from build123d import *

# Parameters (mm, degrees)
SKETCH1_W               = 100
SKETCH1_H               = 40
BOSS_EXTRUDE1_DEPTH     = 5
CUT_EXTRUDE1_DEPTH      = 5
CUT_EXTRUDE2_DEPTH      = 5
CUT_EXTRUDE3_DEPTH      = 5
CUT_EXTRUDE4_DEPTH      = 5
SKETCH3_W               = 70
SKETCH3_H               = 25
BOSS_EXTRUDE2_DEPTH     = 100
FILLET1_R               = 5
FILLET2_R               = 2.5
CUT_EXTRUDE8_DEPTH      = 28.5
FILLET3_R               = 2.5
CUT_EXTRUDE9_DEPTH      = 8.077656227
CUT_EXTRUDE9_DEPTH_BACK = 38.464308309


with BuildPart() as part:
    # Sketch1 → Boss-Extrude1 (new body)
    with BuildSketch(Plane.XY):
        Rectangle(SKETCH1_W, SKETCH1_H)
    extrude(amount=BOSS_EXTRUDE1_DEPTH)

    # Sketch2 → Cut-Extrude1 (cut)
    with BuildSketch(Plane.XY.offset(5)):
        with BuildLine():
            Line((-40.25, 17), (-40.25, -13))
            ThreePointArc((-40.25, -13), (-42.5, -15.25), (-44.75, -13))
            Line((-44.75, -13), (-44.75, 17))
            ThreePointArc((-44.75, 17), (-42.5, 19.25), (-40.25, 17))
        make_face()
    extrude(amount=-CUT_EXTRUDE1_DEPTH, mode=Mode.SUBTRACT)

    # Sketch2_3 → Cut-Extrude2 (cut)
    with BuildSketch(Plane.XY.offset(5)):
        with BuildLine():
            Line((-35, -10.75), (-5, -10.75))
            ThreePointArc((-5, -10.75), (-2.75, -13), (-5, -15.25))
            Line((-5, -15.25), (-35, -15.25))
            ThreePointArc((-35, -15.25), (-37.25, -13), (-35, -10.75))
        make_face()
    extrude(amount=-CUT_EXTRUDE2_DEPTH, mode=Mode.SUBTRACT)

    # Sketch2_4 → Cut-Extrude3 (cut)
    with BuildSketch(Plane.XY.offset(5)):
        with BuildLine():
            Line((5, -10.75), (35, -10.75))
            ThreePointArc((35, -10.75), (37.25, -13), (35, -15.25))
            Line((35, -15.25), (5, -15.25))
            ThreePointArc((5, -15.25), (2.75, -13), (5, -10.75))
        make_face()
    extrude(amount=-CUT_EXTRUDE3_DEPTH, mode=Mode.SUBTRACT)

    # Sketch2_5 → Cut-Extrude4 (cut)
    with BuildSketch(Plane.XY.offset(5)):
        with BuildLine():
            Line((44.75, 17), (44.75, -13))
            ThreePointArc((44.75, -13), (42.5, -15.25), (40.25, -13))
            Line((40.25, -13), (40.25, 17))
            ThreePointArc((40.25, 17), (42.5, 19.25), (44.75, 17))
        make_face()
    extrude(amount=-CUT_EXTRUDE4_DEPTH, mode=Mode.SUBTRACT)

    # Sketch3 → Boss-Extrude2 (add)
    with BuildSketch(Plane.XY.offset(5)):
        with Locations((0, 5)):
            Rectangle(SKETCH3_W, SKETCH3_H)
    extrude(amount=BOSS_EXTRUDE2_DEPTH)

    # Fillet1
    fillet1_edges = [part.edges().sort_by_distance(p)[0] for p in [
        (-50, 20, 2.5),
        (50, 20, 2.5),
        (50, -20, 2.5),
        (-50, -20, 2.5),
    ]]
    fillet(fillet1_edges, radius=FILLET1_R)

    # Fillet2
    fillet2_edges = [part.edges().sort_by_distance(p)[0] for p in [
        (-35, 17.5, 55),
        (-35, -7.5, 55),
        (35, -7.5, 55),
        (35, 17.5, 55),
    ]]
    fillet(fillet2_edges, radius=FILLET2_R)

    # Sketch8 → Cut-Extrude8 (cut, through all)
    with BuildSketch(Plane.XZ.offset(7.5)):
        Polygon((-28.75, 9), (28.75, 9), (28.75, 64.875885604), (0, 89), (-28.75, 64.875885604), align=None)
    extrude(amount=-CUT_EXTRUDE8_DEPTH, mode=Mode.SUBTRACT)

    # Fillet3
    fillet3_edges = [part.edges().sort_by_distance(p)[0] for p in [
        (28.75, 5, 9),
        (-28.75, 5, 9),
        (-28.75, 5, 64.875885604),
        (28.75, 5, 64.875885604),
    ]]
    fillet(fillet3_edges, radius=FILLET3_R)

    # Sketch9 → Cut-Extrude9 (cut, two sides)
    with BuildSketch(Plane(origin=(0, 12.891027114, -0.562834399), x_dir=(-1, 0, 0), z_dir=(0, 0.999048222, -0.043619387))) as cut_extrude9_sk:
        Polygon((17.55, 102.203377148), (22.65, 102.203377148), (22.65, 99.603377148), (-22.65, 99.603377148), (-22.65, 102.203377148), (-17.55, 102.203377148), (-17.55, 108.905331005), (17.55, 108.905331005), align=None)
    extrude(amount=CUT_EXTRUDE9_DEPTH, mode=Mode.SUBTRACT)
    extrude(cut_extrude9_sk.sketch, amount=-CUT_EXTRUDE9_DEPTH_BACK, mode=Mode.SUBTRACT)


solid = part.part
The listing builds one solid part. Answer for the finished solid, in the listing's coordinates (mm). A direction names the side the tool comes from. Round coordinates to 2 decimals unless told otherwise and drop trailing zeros. Write each loop counter-clockwise with the first axis right and the second up, starting at its lowest first coordinate (ties: lowest second). Pieces come first, ordered by that corner, then holes. Notation, with made-up numbers: (28.5, 49.5) - (80.5, 49.5) arc R8 ccw to (80.5, 54.5) - close; hole circle Ø1 at (-7, -23.5). An arc over 180 degrees is marked (long way). Use one line per item in the form item = value. Start each with the question number.
Item 1: A cutting plane is placed at B-B (x = -42.5). Write down the section's boundary in (y, z), plus the area to 3 significant figures.
Item 2: A cutting plane is placed at A-A (y = 10). Give the number of separate pieces and of enclosed holes in the cut face, plus the area to 3 significant figures.
Item 3: A tool of negligible diameter and unlimited length cuts with its end or side. For faces 1 (the flat face through (20.136, 5.175, 102.075)), 2 (the flat face through (14.12, 4.82, 77.15)), 3 (the flat face through (44.75, 2, 3)), 4 (the flat face through (-0.317, 5.175, 99.472)), 5 (the flat face through (-17.55, 5, 103)), from which of +Z, -Z, +X, -X, +Y, -Y can it reach the whole face along a straight path? Write none if from no direction.
Item 4: A cutting plane is placed at C-C (z = 28). Write down the section's boundary in (x, y), plus the area to 3 significant figures.
Item 5: Determine the mould class of faces 6 (the cylindrical face through (42.45, 19.25, 2.54)), 7 (the flat face through (-1, -20, 2)), 8 (the cylindrical face through (48, 19, 3)) for opening direction X: +X half, -X half, draft (parallel to the pull), parting line (faces both ways), or undercut.
Item 6: Find the intervals of material crossed by line 1 (X direction, y = 6, z = 12.5); line 2 (X direction, y = -5, z = 64); line 3 (Z direction, x = 15, y = 13), in increasing order. Write a range as [from, to].
Item 7: A cutting plane is placed at D-D (x = 9.5). Write down the section's boundary in (y, z).
Item 8: Flat-ended cylindrical pins translate along their axes: pin 1 Ø3 at (x, z) = (-28.5, 43) entering from -Y; pin 2 Ø1.8 at (y, z) = (9.5, 101) entering from -X; pin 3 Ø5 at (x, z) = (-9, 78.5) entering from +Y. Find the tip coordinate at first contact, or state that the pin passes through.
The answers:
q1.outline = (-20, 0) - (-15.25, 0) - (-15.25, 5) - (-20, 5) - close; (19.25, 0) - (20, 0) - (20, 5) - (19.25, 5) - close
q1.area = 27.5 mm^2
q2.separate_pieces = 3
q2.enclosed_holes = 1
q2.area = 3,320 mm^2
q3.face_1 = -Y
q3.face_2 = +Y, -Y
q3.face_3 = +Z, -Z
q3.face_4 = +Y
q3.face_5 = +Z, +Y, -Y
q4.outline = (-35, -5) arc R2.5 ccw to (-32.5, -7.5) - (-28.75, -7.5) - (-28.75, 17.5) - (-32.5, 17.5) arc R2.5 ccw to (-35, 15) - close; (28.75, -7.5) - (32.5, -7.5) arc R2.5 ccw to (35, -5) - (35, 15) arc R2.5 ccw to (32.5, 17.5) - (28.75, 17.5) - close
q4.area = 307 mm^2
q5.face_6 = undercut
q5.face_7 = draft
q5.face_8 = +X half
q6.line_1 = [-35, -28.75], [28.75, 35]
q6.line_2 = [-35, -28.73], [28.73, 35]
q6.line_3 = [0, 9], [76.41, 99.13]
q7.outline = (-20, 0) - (-15.25, 0) - (-15.25, 5) - (-20, 5) - close; (-10.75, 0) - (20, 0) - (20, 5) - (17.5, 5) - (17.5, 9) - (-7.5, 9) - (-7.5, 5) - (-10.75, 5) - close; (-7.5, 81.03) - (17.5, 81.03) - (17.5, 98.93) - (-7.5, 100.03) - close
q8.pin_1 = -7.5
q8.pin_2 = -35
q8.pin_3 = 17.5
